from build123d import *

# Parameters (mm, degrees)
SKETCH1_W           = 22
SKETCH1_H           = 56
SKETCH1_W_2         = 15
SKETCH1_H_2         = 15
BOSS_EXTRUDE1_DEPTH = 20
SKETCH2_W           = 15
SKETCH2_H           = 15
SKETCH2_H_2         = 5.5
CUT_EXTRUDE1_DEPTH  = 15.5
FILLET1_R           = 1


with BuildPart() as part:
    # Sketch1 → Boss-Extrude1 (new body)
    with BuildSketch(Plane.XY):
        with Locations((-14.096172604, 14.333947726)):
            Rectangle(SKETCH1_W, SKETCH1_H)
        with Locations((-14.096172604, 31.333947726)):
            Rectangle(SKETCH1_W_2, SKETCH1_H_2, mode=Mode.SUBTRACT)
    extrude(amount=BOSS_EXTRUDE1_DEPTH)

    # Sketch2 → Cut-Extrude1 (cut)
    with BuildSketch(Plane.XY.offset(20)):
        with Locations((-14.096172604, 6.333947726)):
            Rectangle(SKETCH2_W, SKETCH2_H)
        with Locations((-14.096172604, -7.416052274)):
            Rectangle(SKETCH2_W, SKETCH2_H_2)
    extrude(amount=-CUT_EXTRUDE1_DEPTH, mode=Mode.SUBTRACT)

    # Fillet1
    fillet1_edges = [part.edges().sort_by_distance(p)[0] for p in [
        (-3.096172604, 14.333947726, 20),
        (-14.096172604, 42.333947726, 20),
        (-25.096172604, 14.333947726, 20),
        (-14.096172604, 42.333947726, 0),
        (-3.096172604, 14.333947726, 0),
        (-25.096172604, 14.333947726, 0),
        (-25.096172604, 42.333947726, 10),
        (-3.096172604, 42.333947726, 10),
    ]]
    fillet(fillet1_edges, radius=FILLET1_R)


solid = part.part
Can you work these out from the model? Positions are in its coordinate system, mm. A direction names the side the tool comes from. Give positions to 0.01 mm unless a question says otherwise; leave off trailing zeros. Order: outer loops, then holes, each group sorted by start corner. A loop starts at its lowest first (then second) coordinate and runs counter-clockwise, first axis right, second up. Notation, with made-up numbers: M -32,-36 L 7,-36 A20 ccw 7,-11 Z; hole C 1,2 d7. An arc over 180 degrees is marked long. Use one line per item in the form item = value. Start each with the question number.
Item 1: If I drill on line 1 along Y through (x, z) = (-8.75, 11); line 2 along X through (y, z) = (7.5, 14.25); line 3 along Y through (x, z) = (-19, 4), over which ranges is the centre line in solid material (lowest first)?
Item 2: If we section it at D-D (y = -7.5): Write out the boundary of the cut face in (x, z).
Item 3: For faces 5 (the flat face through (-6.596, 31, 10)), 6 (the flat face through (-21.596, -7, 12)), 7 (the flat face through (-14, 8, 0)), which set-ups out of +Z, -Z, +X, -X, +Y, -Y let a thin tool reach every point of the face, with its end or its side?
Item 4: If we section it at C-C (z = 13.5): Write out the boundary of the cut face in (x, y).
Item 5: If we section it at A-A (z = 3.75): Write out the boundary of the cut face in (x, y), then the cut area to 3 significant figures.
Item 6: If we section it at B-B (x = -18.75): Write out the boundary of the cut face in (y, z), then the cut area to 3 significant figures.
Item 7: Will this pin go through, and if not, where does the flat tip stop? pin 1 Ø3 at (x, y) = (-16, -8) entering from +Z.
Item 8: We'd pull the mould along X, two halves only. Please class faces 1 (the flat face through (-3.096, 13, 10)), 2 (the flat face through (-14, 13.834, 12)), 3 (the flat face through (-14, 42.334, 10)), 4 (the flat face through (-6.596, -7, 12)): +X half, -X half, draft (parallel to the pull), parting line (faces both ways), or undercut.
Outcome:
q1.line_1 = -13.67 to -10.17, -4.67 to -1.17, 13.83 to 23.83, 38.83 to 42.33
q1.line_2 = -25.1 to -21.6, -6.6 to -3.1
q1.line_3 = -13.67 to 23.83, 38.83 to 42.33
q2.outline = M -25.1,1 A1 ccw -24.1,0 L -4.1,0 A1 ccw -3.1,1 L -3.1,19 A1 ccw -4.1,20 L -6.6,20 L -6.6,4.5 L -21.6,4.5 L -21.6,20 L -24.1,20 A1 ccw -25.1,19 Z
q3.face_5 = +Z, -Z
q3.face_6 = +Z
q3.face_7 = -Z, +X, -X, +Y, -Y
q4.outline = M -25.1,-13.67 L -3.1,-13.67 L -3.1,41.33 A1 ccw -4.1,42.33 L -24.1,42.33 A1 ccw -25.1,41.33 Z; hole M -21.6,-10.17 L -6.6,-10.17 L -6.6,-4.67 L -21.6,-4.67 Z; hole M -21.6,-1.17 L -6.6,-1.17 L -6.6,13.83 L -21.6,13.83 Z; hole M -21.6,23.83 L -6.6,23.83 L -6.6,38.83 L -21.6,38.83 Z
q5.outline = M -25.1,-13.67 L -3.1,-13.67 L -3.1,41.33 A1 ccw -4.1,42.33 L -24.1,42.33 A1 ccw -25.1,41.33 Z; hole M -21.6,23.83 L -6.6,23.83 L -6.6,38.83 L -21.6,38.83 Z
q5.area = 1,010 mm2
q6.outline = M -13.67,0 L 23.83,0 L 23.83,20 L 13.83,20 L 13.83,4.5 L -1.17,4.5 L -1.17,20 L -4.67,20 L -4.67,4.5 L -10.17,4.5 L -10.17,20 L -13.67,20 Z; M 38.83,0 L 41.33,0 A1 ccw 42.33,1 L 42.33,19 A1 ccw 41.33,20 L 38.83,20 Z
q6.area = 502 mm2
q7.pin_1 = 4.5
q8.face_1 = +X half
q8.face_2 = undercut
q8.face_3 = draft
q8.face_4 = undercut
